from build123d import *

# Parameters (mm, degrees)
CROQUIS1_W                   = 54
CROQUIS1_H                   = 70
CROQUIS1_R                   = 1.5
SALIENTE_EXTRUIR1_DEPTH      = 3
CROQUIS2_R                   = 3
CORTAR_EXTRUIR1_DEPTH        = 1.2
CROQUIS3_W                   = 23.3
CROQUIS3_H                   = 23.3
CROQUIS3_W_2                 = 19.3
CROQUIS3_H_2                 = 19.3
SALIENTE_EXTRUIR2_DEPTH      = 10
CROQUIS4_W                   = 54
CROQUIS4_H                   = 5
SALIENTE_EXTRUIR3_DEPTH      = 75
CROQUIS6_W                   = 54
CROQUIS6_H                   = 20
CORTAR_EXTRUIR2_DEPTH        = 3
CORTAR_EXTRUIR4_DEPTH        = 5
CROQUIS8_W                   = 45
CROQUIS8_H                   = 3.8
CORTAR_EXTRUIR5_DEPTH        = 5
CROQUIS9_W                   = 10.5
CROQUIS9_H                   = 3.7
CORTAR_EXTRUIR6_DEPTH        = 3
SALIENTE_EXTRUIR4_DEPTH      = 8
SALIENTE_EXTRUIR4_DEPTH_BACK = 4
SALIENTE_EXTRUIR5_DEPTH      = 20
CROQUIS12_W                  = 9
CROQUIS12_H                  = 7
CORTAR_EXTRUIR7_DEPTH        = 4
CROQUIS13_W                  = 40
CROQUIS13_H                  = 13
SALIENTE_EXTRUIR6_DEPTH      = 4
CROQUIS16_W                  = 9
CROQUIS16_H                  = 3.2
CORTAR_EXTRUIR9_DEPTH        = 4
CROQUIS17_W                  = 20
CROQUIS17_H                  = 32
SALIENTE_EXTRUIR7_DEPTH      = 3


with BuildPart() as part:
    # Croquis1 → Saliente-Extruir1 (new body)
    with BuildSketch(Plane.XY):
        Rectangle(CROQUIS1_W, CROQUIS1_H)
        with Locations((-7.5, 0)):
            Circle(CROQUIS1_R, mode=Mode.SUBTRACT)
        with Locations(Location((7.5, 0, 0), (0, 0, 180))):
            Circle(CROQUIS1_R, mode=Mode.SUBTRACT)
    extrude(amount=SALIENTE_EXTRUIR1_DEPTH)

    # Croquis2 → Cortar-Extruir1 (cut)
    with BuildSketch(Plane.XY.offset(3)):
        with Locations((-7.5, 0)):
            Circle(CROQUIS2_R)
        with Locations(Location((7.5, 0, 0), (0, 0, 180))):
            Circle(CROQUIS2_R)
    extrude(amount=-CORTAR_EXTRUIR1_DEPTH, mode=Mode.SUBTRACT)

    # Croquis3 → Saliente-Extruir2 (add)
    with BuildSketch(Plane.XY.offset(3)):
        with Locations((0, 16.35)):
            Rectangle(CROQUIS3_W, CROQUIS3_H)
        with Locations((0, 16.35)):
            Rectangle(CROQUIS3_W_2, CROQUIS3_H_2, mode=Mode.SUBTRACT)
    extrude(amount=SALIENTE_EXTRUIR2_DEPTH)

    # Croquis4 → Saliente-Extruir3 (add)
    with BuildSketch(Plane(origin=(0, 0, 0), x_dir=(-1, 0, 0), z_dir=(0, 0, -1))):
        with Locations((0, 32.5)):
            Rectangle(CROQUIS4_W, CROQUIS4_H)
    extrude(amount=SALIENTE_EXTRUIR3_DEPTH)

    # Croquis6 → Cortar-Extruir2 (cut)
    with BuildSketch(Plane(origin=(0, 0, 0), x_dir=(-1, 0, 0), z_dir=(0, 0, -1))):
        with Locations((0, -25)):
            Rectangle(CROQUIS6_W, CROQUIS6_H)
    extrude(amount=-CORTAR_EXTRUIR2_DEPTH, mode=Mode.SUBTRACT)

    # Croquis7 → Cortar-Extruir4 (cut)
    with BuildSketch(Plane(origin=(0, 35, 0), x_dir=(1, 0, 0), z_dir=(0, 1, 0))):
        Polygon((-27, 75), (-21, 75), (-23.25, 25), (-27, 25), align=None)
        Polygon((23.25, 25), (27, 25), (27, 75), (21, 75), align=None)
    extrude(amount=-CORTAR_EXTRUIR4_DEPTH, mode=Mode.SUBTRACT)

    # Croquis8 → Cortar-Extruir5 (cut)
    with BuildSketch(Plane(origin=(0, 35, 0), x_dir=(1, 0, 0), z_dir=(0, 1, 0))):
        with Locations((0, 13.816893204)):
            Rectangle(CROQUIS8_W, CROQUIS8_H)
    extrude(amount=-CORTAR_EXTRUIR5_DEPTH, mode=Mode.SUBTRACT)

    # Croquis9 → Cortar-Extruir6 (cut)
    with BuildSketch(Plane.XY.offset(3)):
        with Locations((4.4, 24.15)):
            Rectangle(CROQUIS9_W, CROQUIS9_H)
        with BuildLine():
            Line((5.5, 6.7), (-5.5, 6.7))
            ThreePointArc((-5.5, 6.7), (0, 12.2), (5.5, 6.7))
        make_face()
    extrude(amount=-CORTAR_EXTRUIR6_DEPTH, mode=Mode.SUBTRACT)

    # Croquis10 → Saliente-Extruir4 (add, two sides: drawn at the far end of the back side and taken through both)
    with BuildSketch(Plane(origin=(0, 35, 0), x_dir=(1, 0, 0), z_dir=(0, 1, 0)).offset(-SALIENTE_EXTRUIR4_DEPTH_BACK)):
        Polygon((-21, 75), (-27, 75), (-27, 35), (-22.8, 35), align=None)
        Polygon((27, 35), (22.8, 35), (21, 75), (27, 75), align=None)
    extrude(amount=SALIENTE_EXTRUIR4_DEPTH + SALIENTE_EXTRUIR4_DEPTH_BACK)

    # Croquis11 → Saliente-Extruir5 (add)
    with BuildSketch(Plane(origin=(27, 0, 0), x_dir=(0, 0, -1), z_dir=(1, 0, 0))):
        Polygon((35, 43), (39, 43), (39, 34), (71, 34), (71, 43), (75, 43), (75, 30), (35, 30), align=None)
    extrude(amount=SALIENTE_EXTRUIR5_DEPTH)

    # Croquis12 → Cortar-Extruir7 (cut)
    with BuildSketch(Plane(origin=(0, 0, -75), x_dir=(-1, 0, 0), z_dir=(0, 0, -1))):
        with Locations((-42.5, 37.5)):
            Rectangle(CROQUIS12_W, CROQUIS12_H)
    extrude(amount=-CORTAR_EXTRUIR7_DEPTH, mode=Mode.SUBTRACT)

    # Croquis13 → Saliente-Extruir6 (add)
    with BuildSketch(Plane(origin=(47, 0, 0), x_dir=(0, 0, -1), z_dir=(1, 0, 0))):
        with Locations((55, 36.5)):
            Rectangle(CROQUIS13_W, CROQUIS13_H)
    extrude(amount=SALIENTE_EXTRUIR6_DEPTH)

    # Croquis16 → Cortar-Extruir9 (cut)
    with BuildSketch(Plane.XY.offset(-35)):
        with Locations((41, 39.4)):
            Rectangle(CROQUIS16_W, CROQUIS16_H)
    extrude(amount=-CORTAR_EXTRUIR9_DEPTH, mode=Mode.SUBTRACT)

    # Croquis17 → Saliente-Extruir7 (add)
    with BuildSketch(Plane(origin=(0, 43, 0), x_dir=(1, 0, 0), z_dir=(0, 1, 0))):
        Polygon((21, 75), (51, 75), (51, 35), (22.8, 35), align=None)
        with Locations((37, 55)):
            Rectangle(CROQUIS17_W, CROQUIS17_H, mode=Mode.SUBTRACT)
    extrude(amount=SALIENTE_EXTRUIR7_DEPTH)


solid = part.part
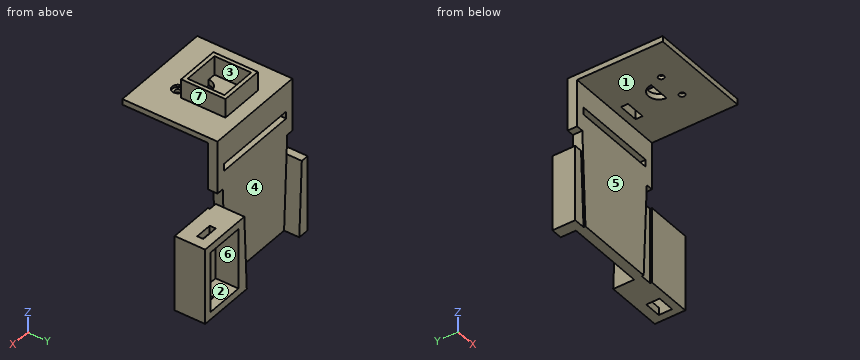
Model file for the job. Use its own axes, mm. Face numbers are marked on the shaded views. A direction names the side the tool comes from. Give positions to 0.01 mm unless a question says otherwise; leave off trailing zeros. Loops run counter-clockwise (first coordinate to the right, second up) from the corner with the lowest first, then second, coordinate; pieces in that order, holes last.
Item 1: Slice it at B-B (y = 0). Write the cut outline in (x, z).
Check values:
outline: (-27, 0) - (-9, 0) - (-9, 1.8) - (-10.5, 1.8) - (-10.5, 3) - (-27, 3) - close; (-6, 0) - (6, 0) - (6, 1.8) - (4.5, 1.8) - (4.5, 3) - (-4.5, 3) - (-4.5, 1.8) - (-6, 1.8) - close; (9, 0) - (27, 0) - (27, 3) - (10.5, 3) - (10.5, 1.8) - (9, 1.8) - close
Item 2: Slice it at C-C (x = 35). Write the cut outline in (y, z), plus the area to 3 significant figures.
Check values:
outline: (30, -75) - (46, -75) - (46, -71) - (34, -71) - (34, -39) - (46, -39) - (46, -35) - (30, -35) - close
area: 256 mm2
Item 3: Slice it at D-D (z = -50.5). Write the cut outline in (x, y).
Check values:
outline: (-27, 31) - (-22.1, 31) - (-22.1, 30) - (22.1, 30) - (22.1, 31) - (27, 31) - (27, 30) - (51, 30) - (51, 46) - (47, 46) - (47, 34) - (27, 34) - (27, 46) - (22.1, 46) - (22.1, 35) - (-22.1, 35) - (-22.1, 43) - (-27, 43) - close
Item 4: Drop flat-ended pins along their axis: P1, Ø4.5, axis at x = 42, z = -37, coming from the -Y side; P2, Ø1.9, axis at y = 33, z = -14.5, coming from the +X side; P3, Ø1, axis at x = 7, z = -5.5, coming from the +Y side; P4, Ø11, axis at x = -3.5, z = 7, coming from the -Y side. Give the stop position or say it passes through.
Check values:
P1: stops at y = 30
P2: stops at x = 27
P3: stops at y = 35
P4: stops at y = -15
Item 5: Drill centre lines: line 1 along X through (y, z) = (17, 5); line 2 along Z through (x, y) = (45, 41.5); line 3 along Y through (x, z) = (-7.5, 1.2). Where is each one in solid material? Low to high.
Check values:
line 1: x = -11.65 to -9.65, 9.65 to 11.65
line 2: z = -75 to -71, -39 to -35
line 3: y = -15 to -1.5, 1.5 to 35
Item 6: Which spindle directions (+Z, -Z, +X, -X, +Y, -Y) get a long thin tool onto all of the face, cutting with end or side? Do the marked faces 1, 2 and 3. Say none if no direction does.
Check values:
face 1: -Z, +X, -X, -Y
face 2: +Y
face 3: +Z
Item 7: Mould opens along X. For the marked faces 4, 5, 6 and 7 say: +X half, -X half, draft (parallel to the pull), parting line (faces both ways), or undercut.
Check values:
face 4: undercut
face 5: draft
face 6: undercut
face 7: +X half
Item 8: Slice it at A-A (x = -7.5). Write the cut outline in (y, z), plus the area to 3 significant figures.
Check values:
outline: (-15, 0) - (-1.5, 0) - (-1.5, 1.8) - (-3, 1.8) - (-3, 3) - (-15, 3) - close; (1.5, 0) - (30, 0) - (30, -11.92) - (35, -11.92) - (35, 3) - (28, 3) - (28, 13) - (26, 13) - (26, 3) - (6.7, 3) - (6.7, 13) - (4.7, 13) - (4.7, 3) - (3, 3) - (3, 1.8) - (1.5, 1.8) - close; (30, -75) - (35, -75) - (35, -15.72) - (30, -15.72) - close
area: 533 mm2
